from build123d import *

# Parameters (mm, degrees)
ESQUISSE1_W             = 35
ESQUISSE1_H             = 35
BOSS_EXTRU_1_DEPTH      = 3
ESQUISSE2_W             = 35
ESQUISSE2_H             = 2.3
BOSS_EXTRU_2_DEPTH      = 5.2
ESQUISSE3_R             = 1.25
ENL_V_MAT_EXTRU_1_DEPTH = 45
D_GAGEMENT_M2_51_D      = 2.9
D_GAGEMENT_M2_52_D      = 2.9
D_GAGEMENT_M2_53_D      = 2.9
CONG_1_R                = 1


with BuildPart() as part:
    # Esquisse1 → Boss.-Extru.1 (new body)
    with BuildSketch(Plane.XY):
        with Locations((-2.901069519, 5.614973262)):
            Rectangle(ESQUISSE1_W, ESQUISSE1_H)
    extrude(amount=BOSS_EXTRU_1_DEPTH)

    # Esquisse2 → Boss.-Extru.2 (add)
    with BuildSketch(Plane(origin=(0, 0, 0), x_dir=(-1, 0, 0), z_dir=(0, 0, -1))):
        with Locations((2.901069519, 21.964973262)):
            Rectangle(ESQUISSE2_W, ESQUISSE2_H)
        with Locations((2.901069519, -10.735026738)):
            Rectangle(ESQUISSE2_W, ESQUISSE2_H)
    extrude(amount=BOSS_EXTRU_2_DEPTH)

    # Esquisse3 → Enlèv. mat.-Extru.1 (cut)
    with BuildSketch(Plane(origin=(0, 23.114973262, 0), x_dir=(1, 0, 0), z_dir=(0, 1, 0))):
        with Locations(Location((-11.401069519, 2.8, 0), (0, 0, 270))):
            Circle(ESQUISSE3_R)
        with Locations(Location((5.598930481, 2.8, 0), (0, 0, 270))):
            Circle(ESQUISSE3_R)
    extrude(amount=-ENL_V_MAT_EXTRU_1_DEPTH, mode=Mode.SUBTRACT)

    # Dégagement M2.51 (through all)
    with Locations(Plane(origin=(0, 23.114973262, 0), x_dir=(1, 0, 0), z_dir=(0, 1, 0))):
        with Locations((-11.401069519, 2.8), (5.598930481, 2.8)):
            Hole(D_GAGEMENT_M2_51_D / 2)

    # Dégagement M2.52 (through all)
    with Locations(Plane(origin=(0, -11.885026738, 0), x_dir=(-1, 0, 0), z_dir=(0, -1, 0))):
        with Locations((11.401069519, 2.8), (-5.598930481, 2.8)):
            Hole(D_GAGEMENT_M2_52_D / 2)

    # Dégagement M2.53 (through all)
    with Locations(Plane(origin=(0, 0, 0), x_dir=(-1, 0, 0), z_dir=(0, 0, -1))):
        with Locations((-4.848930481, 13.364973262), (10.651069519, 13.364973262), (10.651069519, -2.135026738), (-4.848930481, -2.135026738)):
            Hole(D_GAGEMENT_M2_53_D / 2)

    # Congé1
    # the kernel refuses this fillet: 1 mm, written as the material it takes off along each edge
    with BuildSketch(Plane(origin=(13.598930481, 22.114973262, 2), x_dir=(0, 0, 1), z_dir=(0, 1, 0))) as cong_1_piece_1_section:
        Polygon((0, 0), (CONG_1_R, 0), (CONG_1_R, CONG_1_R), (0, CONG_1_R), align=None)
    cong_1_piece_1 = extrude(amount=CONG_1_R, mode=Mode.PRIVATE)
    cong_1_piece_1 = cong_1_piece_1 - Plane(origin=(13.598930481, 22.114973262, 2), x_dir=(-0.7071067811865475, 0, -0.7071067811865475), z_dir=(0, 1, 0)) * Sphere(CONG_1_R, mode=Mode.PRIVATE)
    add(cong_1_piece_1, mode=Mode.SUBTRACT)
    with BuildSketch(Plane(origin=(-19.401069519, 22.114973262, 2), x_dir=(0, 0, 1), z_dir=(0, 1, 0))) as cong_1_piece_2_section:
        Polygon((0, 0), (CONG_1_R, 0), (CONG_1_R, -CONG_1_R), (0, -CONG_1_R), align=None)
    cong_1_piece_2 = extrude(amount=CONG_1_R, mode=Mode.PRIVATE)
    cong_1_piece_2 = cong_1_piece_2 - Plane(origin=(-19.401069519, 22.114973262, 2), x_dir=(0.7071067811865475, 0, -0.7071067811865475), z_dir=(0, 1, 0)) * Sphere(CONG_1_R, mode=Mode.PRIVATE)
    add(cong_1_piece_2, mode=Mode.SUBTRACT)
    with BuildSketch(Plane(origin=(-19.401069519, -10.885026738, 2), x_dir=(-1, 0, 0), z_dir=(0, 0, 1))) as cong_1_piece_3_section:
        Polygon((0, 0), (CONG_1_R, 0), (CONG_1_R, CONG_1_R), (0, CONG_1_R), align=None)
    cong_1_piece_3 = extrude(amount=CONG_1_R, mode=Mode.PRIVATE)
    cong_1_piece_3 = cong_1_piece_3 - Plane(origin=(-19.401069519, -10.885026738, 2), x_dir=(0.7071067811865475, 0.7071067811865477, 0), z_dir=(0, 0, 1)) * Sphere(CONG_1_R, mode=Mode.PRIVATE)
    add(cong_1_piece_3, mode=Mode.SUBTRACT)
    with BuildSketch(Plane(origin=(14.598930481, 22.114973262, 3), x_dir=(-1, 0, 0), z_dir=(0, -1, 0)), Plane(origin=(17.098930481, -11.885026738, 3), x_dir=(0, 1, 0), z_dir=(-1, 0, 0))) as cong_1_piece_4:
        with BuildLine():
            CenterArc((CONG_1_R, CONG_1_R), CONG_1_R, 180, 90)
            Line((0, CONG_1_R), (0, 0))
            Line((0, 0), (CONG_1_R, 0))
        make_face()
    extrude(amount=36.5, mode=Mode.SUBTRACT)
    with BuildSketch(Plane(origin=(-19.401069519, 23.114973262, 3), x_dir=(0, 0, -1), z_dir=(1, 0, 0))) as cong_1_piece_5:
        with BuildLine():
            CenterArc((CONG_1_R, -CONG_1_R), CONG_1_R, 90, 90)
            Line((0, -CONG_1_R), (0, 0))
            Line((0, 0), (CONG_1_R, 0))
        make_face()
    extrude(amount=33, mode=Mode.SUBTRACT)
    with BuildSketch(Plane(origin=(17.098930481, -11.885026738, -5.2), x_dir=(0, 0, 1), z_dir=(-1, 0, 0))) as cong_1_piece_6:
        with BuildLine():
            CenterArc((CONG_1_R, CONG_1_R), CONG_1_R, 180, 90)
            Line((0, CONG_1_R), (0, 0))
            Line((0, 0), (CONG_1_R, 0))
        make_face()
    extrude(amount=40, mode=Mode.SUBTRACT)
    with BuildSketch(Plane(origin=(-20.401069519, -10.885026738, 3), x_dir=(1, 0, 0), z_dir=(0, 1, 0))) as cong_1_piece_7:
        with BuildLine():
            CenterArc((CONG_1_R, CONG_1_R), CONG_1_R, 180, 90)
            Line((0, CONG_1_R), (0, 0))
            Line((0, 0), (CONG_1_R, 0))
        make_face()
    extrude(amount=33, mode=Mode.SUBTRACT)
    with BuildSketch(Plane(origin=(-20.401069519, 23.114973262, -7.7), x_dir=(1, 0, 0), z_dir=(0, 0, 1)), Plane(origin=(14.598930481, 23.114973262, 2), x_dir=(-1, 0, 0), z_dir=(0, 0, -1)), Plane(origin=(-20.401069519, -11.885026738, -7.7), x_dir=(0, 1, 0), z_dir=(0, 0, 1))) as cong_1_piece_8:
        with BuildLine():
            CenterArc((CONG_1_R, -CONG_1_R), CONG_1_R, 90, 90)
            Line((0, -CONG_1_R), (0, 0))
            Line((0, 0), (CONG_1_R, 0))
        make_face()
    extrude(amount=9.7, mode=Mode.SUBTRACT)


solid = part.part
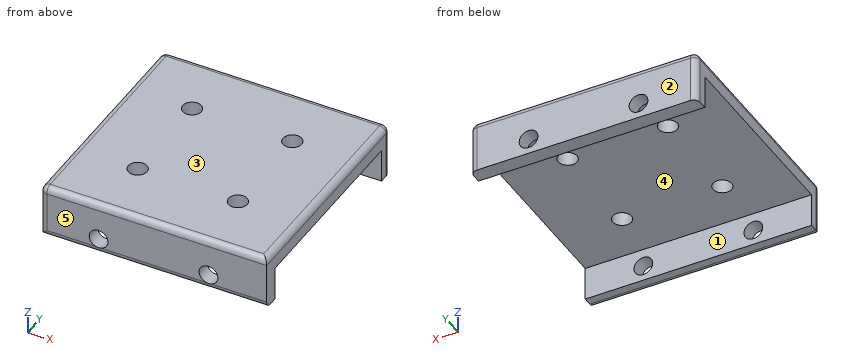
For this review, take the finished solid that the model builds, in its own axes (mm). Face numbers are marked on the shaded views. A direction names the side the tool comes from. Coordinates: 2 decimals unless noted, no trailing zeros. Loops run counter-clockwise (first coordinate to the right, second up) from the corner with the lowest first, then second, coordinate; pieces in that order, holes last. Notation, with made-up numbers: (76.5, 71) -> (134.5, 71) arc R28 cw to (134.5, 89) -> close; hole circle Ø5 at (73, 72.25). An arc over 180 degrees is marked (long way). Write each question's results on one line, items separated by ' | '.
Q1. To check wall thickness, follow line 1 along X through (y, z) = (-10, -1.5); line 2 along Y through (x, z) = (3, -3.5); line 3 along Z through (x, y) = (-3, 7.5). State the ranges of each line that lie inside material, in increasing order. Write a range as [from, to].
Taken from the geometry:
line 1: [-20.4, -12.04], [-10.76, 4.96], [6.24, 14.6] | line 2: [-11.89, -9.59], [20.81, 23.11] | line 3: [0, 3]
Q2. Mouldability with a two-part tool opening along Y and no side actions: class the marked faces 3, 4 and 5 as +Y half, -Y half, draft (parallel to the pull), parting line (faces both ways), or undercut.
Taken from the geometry:
face 3: draft | face 4: undercut | face 5: -Y half
Q3. Add section A-A, the plane z = -2.8. State the section outline as (x, y) points.
Taken from the geometry:
outline: (-20.4, -10.89) arc R1 ccw to (-19.4, -11.89) -> (-12.85, -11.89) -> (-12.85, -9.59) -> (-20.4, -9.59) -> close; (-20.4, 20.81) -> (-12.85, 20.81) -> (-12.85, 23.11) -> (-19.4, 23.11) arc R1 ccw to (-20.4, 22.11) -> close; (-9.95, -11.89) -> (4.15, -11.89) -> (4.15, -9.59) -> (-9.95, -9.59) -> close; (-9.95, 20.81) -> (4.15, 20.81) -> (4.15, 23.11) -> (-9.95, 23.11) -> close; (7.05, -11.89) -> (14.6, -11.89) -> (14.6, -9.59) -> (7.05, -9.59) -> close; (7.05, 20.81) -> (14.6, 20.81) -> (14.6, 22.11) arc R1 ccw to (13.6, 23.11) -> (7.05, 23.11) -> close
Q4. Add section B-B, the plane x = -5.5. State the section outline as (y, z) points.
Taken from the geometry:
outline: (-11.89, -4.2) arc R1 ccw to (-10.89, -5.2) -> (-9.59, -5.2) -> (-9.59, 0) -> (20.81, 0) -> (20.81, -5.2) -> (23.11, -5.2) -> (23.11, 2) arc R1 ccw to (22.11, 3) -> (-10.89, 3) arc R1 ccw to (-11.89, 2) -> close
Q5. Machinability: for the marked faces 1 and 2, which of the approach directions +Z, -Z, +X, -X, +Y, -Y give a long, thin tool a straight path to every point of the face, cutting with its end or side? Answer none if there is none.
Taken from the geometry:
face 1: -Z, +X, -X | face 2: +Z, -Z, +X, -X, +Y
Q6. For pin 1 Ø12 at (x, y) = (6.5, 3.5) entering from -Z, flat-tipped, find the tip position at first contact; note if it passes through.
Taken from the geometry:
pin 1: z = 0
Q7. Add section C-C, the plane y = -8. State the section outline as (x, z) points.
Taken from the geometry:
outline: (-20.4, 0) -> (14.6, 0) -> (14.6, 2) arc R1 ccw to (13.6, 3) -> (-19.4, 3) arc R1 ccw to (-20.4, 2) -> close
